Part print with two shaded views. Sizes in mm from the minimum x, y, z corner. A direction names the side the tool comes from. Round coordinates to 2 decimals unless told otherwise and drop trailing zeros. Write each loop counter-clockwise with the first axis right and the second up, starting at its lowest first coordinate (ties: lowest second). Pieces come first, ordered by that corner, then holes. Notation, with made-up numbers: (-7.5, 26.25) -> (17.5, 26.25) arc R15 ccw to (17.5, 42.25) -> close; hole circle Ø7 at (50, 18). An arc over 180 degrees is marked (long way). Return JSON: item names as keys, results as strings.
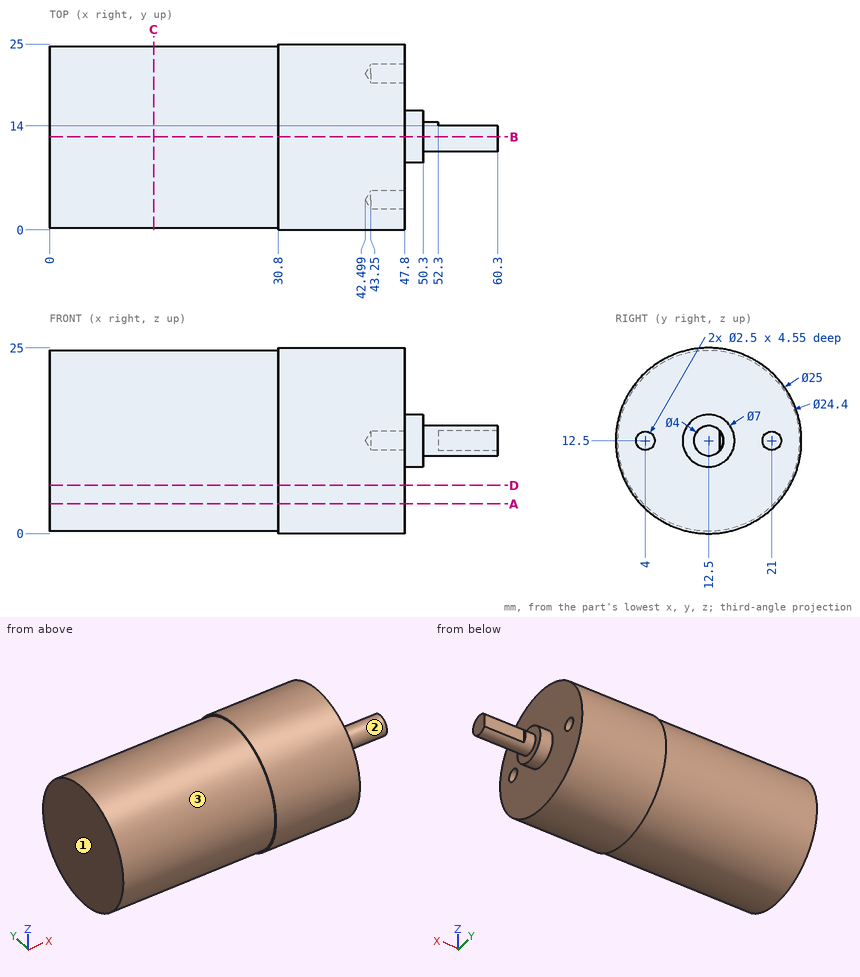
Q1. 3-axis set-ups, long thin cutter, end or side, ignore diameter. For the marked faces 1, 2 and 3: which of +Z, -Z, +X, -X, +Y, -Y reach the whole face in a straight line?
Verdict:
{"face 1": "+Z, -Z, -X, +Y, -Y", "face 2": "+X", "face 3": "-X"}
Q2. Saw through at B-B on y = 12.5. List the corners of the cut face in (x, z).
Verdict:
{"outline": "(0, 0.3) -> (30.8, 0.3) -> (30.8, 0) -> (47.8, 0) -> (47.8, 9) -> (50.3, 9) -> (50.3, 10.5) -> (60.3, 10.5) -> (60.3, 14.5) -> (50.3, 14.5) -> (50.3, 16) -> (47.8, 16) -> (47.8, 25) -> (30.8, 25) -> (30.8, 24.7) -> (0, 24.7) -> close"}
Q3. Saw through at C-C on x = 14. List the corners of the cut face in (y, z), then the cut area to 3 significant figures.
Verdict:
{"outline": "circle Ø24.4 at (12.5, 12.5)", "area": "468 mm²"}
Q4. Saw through at D-D on z = 6.5. List the corners of the cut face in (x, y).
Verdict:
{"outline": "(0, 1.88) -> (30.8, 1.88) -> (30.8, 1.53) -> (47.8, 1.53) -> (47.8, 23.47) -> (30.8, 23.47) -> (30.8, 23.12) -> (0, 23.12) -> close"}
Q5. Pin check, flat tips, straight feed: pin 1 Ø6 at (y, z) = (4, 15) entering from +X; pin 2 Ø1.3 at (x, z) = (56.5, 13) entering from +Y; pin 3 Ø10 at (x, z) = (12, 10) entering from +Y. Stop position of each tip, or through.
Verdict:
{"pin 1": "stops at x = 47.8", "pin 2": "stops at y = 14", "pin 3": "stops at y = 24.7"}
Q6. Wall check: L1, parallel to Y at x = 44.45, z = 12.5; L2, parallel to X at y = 23.25, z = 8.5; L3, parallel to X at y = 12.25, z = 15.25. Give the ranges that are in metal, low to high.
Verdict:
{"L1": "y = 0 to 2.75, 5.25 to 19.75, 22.25 to 25", "L2": "x = 0 to 47.8", "L3": "x = 0 to 50.3"}
Q7. Saw through at A-A on z = 4. List the corners of the cut face in (x, y) (1 decimal).
Verdict:
{"outline": "(0, 3.7) -> (30.8, 3.7) -> (30.8, 3.3) -> (47.8, 3.3) -> (47.8, 21.7) -> (30.8, 21.7) -> (30.8, 21.3) -> (0, 21.3) -> close"}
